For this review, take the finished solid that the model builds, in its own axes (mm). Face numbers are marked on the shaded views. A direction names the side the tool comes from. Round coordinates to 2 decimals unless told otherwise and drop trailing zeros. Write each loop counter-clockwise with the first axis right and the second up, starting at its lowest first coordinate (ties: lowest second). Pieces come first, ordered by that corner, then holes. Notation, with made-up numbers: (14.25, -18) -> (23.25, -18) arc R6 cw to (23.25, -7) -> close; hole circle Ø2 at (-24, -4). An arc over 180 degrees is marked (long way). Answer in a Markdown table with one row per item.
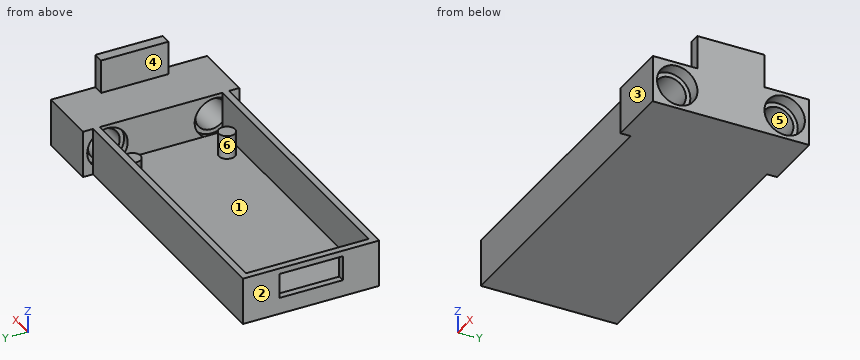
from build123d import *

# Parameters (mm, degrees)
SKETCH1_W              = 39
SKETCH1_H              = 20.2
BOSS_EXTRUDE1_DEPTH    = 7
SKETCH2_W              = 38
SKETCH2_H              = 18.2
CUT_EXTRUDE1_DEPTH     = 6
SKETCH3_R              = 1.2
SPUNT_DEPTH            = 3.5
SKETCH5_W              = 3.7
SKETCH5_H              = 9.4
USBC_DEPTH             = 22
ROZSIRENI_DRZAKU_DEPTH = 3
SKETCH7_W              = 7
SKETCH7_H              = 23.2
DRZAK_DEPTH            = 9
SKETCH8_R              = 2.35
ZAKLADNI_DIRA_DEPTH    = 9
SKETCH9_R              = 3
CUT_EXTRUDE4_DEPTH     = 2
SKETCH11_R             = 3
CUT_EXTRUDE5_DEPTH     = 1
SKETCH10_W             = 1.6
SKETCH10_H             = 10
PODSTAVA_DEPTH         = 5


with BuildPart() as part:
    # Sketch1 → Boss-Extrude1 (new body)
    with BuildSketch(Plane.XY):
        Rectangle(SKETCH1_W, SKETCH1_H)
    extrude(amount=BOSS_EXTRUDE1_DEPTH)

    # Sketch2 → Cut-Extrude1 (cut)
    with BuildSketch(Plane.XY.offset(7)):
        with Locations((0.5, 0)):
            Rectangle(SKETCH2_W, SKETCH2_H)
    extrude(amount=-CUT_EXTRUDE1_DEPTH, mode=Mode.SUBTRACT)

    # Sketch3 → spunt (add)
    with BuildSketch(Plane.XY.offset(1)):
        with Locations((17.3, -7)):
            Circle(SKETCH3_R)
        with Locations((17.3, 7)):
            Circle(SKETCH3_R)
    extrude(amount=SPUNT_DEPTH)

    # Sketch5 → usbc (cut)
    with BuildSketch(Plane(origin=(-18.5, 0, 0), x_dir=(0, 0, -1), z_dir=(1, 0, 0))):
        with Locations((-4.3, 0)):
            Rectangle(SKETCH5_W, SKETCH5_H)
    extrude(amount=-USBC_DEPTH, mode=Mode.SUBTRACT)

    # Sketch6 → rozsireni drzaku (add)
    with BuildSketch(Plane(origin=(19.5, 0, 0), x_dir=(0, 0, -1), z_dir=(1, 0, 0))):
        Polygon((-7, -10.1), (0, -10.1), (0, 10.1), (-7, 10.1), (-7, 9.1), (-1, 9.1), (-1, -9.1), (-7, -9.1), align=None)
    extrude(amount=ROZSIRENI_DRZAKU_DEPTH)

    # Sketch7 → drzak (add)
    with BuildSketch(Plane(origin=(22.5, 0, 0), x_dir=(0, 0, -1), z_dir=(1, 0, 0))):
        with Locations((-3.5, 0)):
            Rectangle(SKETCH7_W, SKETCH7_H)
    extrude(amount=DRZAK_DEPTH)

    # Sketch8 → zakladni dira (cut)
    with BuildSketch(Plane(origin=(31.5, 0, 0), x_dir=(0, 0, -1), z_dir=(1, 0, 0))):
        with Locations((-3.5, 7.97)):
            Circle(SKETCH8_R)
        with Locations((-3.5, -7.97)):
            Circle(SKETCH8_R)
    extrude(amount=-ZAKLADNI_DIRA_DEPTH, mode=Mode.SUBTRACT)

    # Sketch9 → Cut-Extrude4 (cut)
    with BuildSketch(Plane(origin=(31.5, 0, 0), x_dir=(0, 0, -1), z_dir=(1, 0, 0))):
        with Locations((-3.5, 7.97)):
            Circle(SKETCH9_R)
        with Locations((-3.5, -7.97)):
            Circle(SKETCH9_R)
    extrude(amount=-CUT_EXTRUDE4_DEPTH, mode=Mode.SUBTRACT)

    # Sketch11 → Cut-Extrude5 (cut)
    with BuildSketch(Plane.ZY.offset(-22.5)):
        with Locations((3.5, -7.97)):
            Circle(SKETCH11_R)
        with Locations((3.5, 7.97)):
            Circle(SKETCH11_R)
    extrude(amount=-CUT_EXTRUDE5_DEPTH, mode=Mode.SUBTRACT)

    # Sketch10 → podstava (add)
    with BuildSketch(Plane.XY.offset(7)):
        with Locations((30.7, 0)):
            Rectangle(SKETCH10_W, SKETCH10_H)
    extrude(amount=PODSTAVA_DEPTH)


solid = part.part
1) For the marked faces 4, 5 and 6, list the 3-axis set-ups (+Z, -Z, +X, -X, +Y, -Y) from which the entire face can be reached by the end or side of a thin tool; tool diameter is ignored.
Solved:
| item | result |
|---|---|
| face 4 | +Z, -X, +Y, -Y |
| face 5 | +X |
| face 6 | +Z |
2) Consider section B-B on x = 17.3. State the section outline as (y, z) points, then the cut area to 3 significant figures.
Solved:
| item | result |
|---|---|
| outline | (-10.1, 0) -> (10.1, 0) -> (10.1, 7) -> (9.1, 7) -> (9.1, 1) -> (8.2, 1) -> (8.2, 4.5) -> (5.8, 4.5) -> (5.8, 1) -> (-5.8, 1) -> (-5.8, 4.5) -> (-8.2, 4.5) -> (-8.2, 1) -> (-9.1, 1) -> (-9.1, 7) -> (-10.1, 7) -> close |
| area | 49.0 mm² |
3) For line 1 (Y direction, x = 26.2, z = 3.5); line 2 (X direction, y = 4.25, z = 1.25); line 3 (Z direction, x = 22.8, y = -7.97), list the stretches that pass through material, from the lowest coordinate up. Write a range as [from, to].
Solved:
| item | result |
|---|---|
| line 1 | [-11.6, -10.32], [-5.62, 5.62], [10.32, 11.6] |
| line 2 | [-19.5, -18.5], [22.5, 31.5] |
| line 3 | [0, 0.5], [6.5, 7] |
4) Consider section C-C on z = 3.5. State how many separate pieces and enclosed holes the cut face has, then the cut area to 3 significant figures.
Solved:
| item | result |
|---|---|
| separate pieces | 7 |
| enclosed holes | 0 |
| area | 218 mm² |
5) Mouldability with a two-part tool opening along X and no side actions: class the marked faces 1, 2 and 3 as pulls with the +X half, pulls with the -X half, needs draft (parallel to the pull), parting line crosses it, or undercut.
Solved:
| item | result |
|---|---|
| face 1 | undercut |
| face 2 | pulls with the -X half |
| face 3 | needs draft |
6) Consider section D-D on y = 7. State the section outline as (x, z) points, then the cut area to 3 significant figures.
Solved:
| item | result |
|---|---|
| outline | (-19.5, 0) -> (31.5, 0) -> (31.5, 0.66) -> (29.5, 0.66) -> (29.5, 1.36) -> (23.5, 1.36) -> (23.5, 0.66) -> (22.5, 0.66) -> (22.5, 1) -> (18.5, 1) -> (18.5, 4.5) -> (16.1, 4.5) -> (16.1, 1) -> (-18.5, 1) -> (-18.5, 7) -> (-19.5, 7) -> close; (22.5, 6.34) -> (23.5, 6.34) -> (23.5, 5.64) -> (29.5, 5.64) -> (29.5, 6.34) -> (31.5, 6.34) -> (31.5, 7) -> (22.5, 7) -> close |
| area | 76.7 mm² |
7) Consider section A-A on y = -0.75. State the section outline as (x, z) points.
Solved:
| item | result |
|---|---|
| outline | (-19.5, 0) -> (31.5, 0) -> (31.5, 12) -> (29.9, 12) -> (29.9, 7) -> (22.5, 7) -> (22.5, 1) -> (-18.5, 1) -> (-18.5, 2.45) -> (-19.5, 2.45) -> close; (-19.5, 6.15) -> (-18.5, 6.15) -> (-18.5, 7) -> (-19.5, 7) -> close |
8) Clearance check with flat-ended pins moving along their axes: pin 1 Ø5 at (x, y) = (-7.5, 6.5) entering from +Z; pin 2 Ø1.2 at (x, y) = (17, 7.5) entering from +Z; pin 3 Ø3 at (x, z) = (3, 5) entering from -Y. State where each tip first meets the part, or that it passes through.
Solved:
| item | result |
|---|---|
| pin 1 | z = 1 |
| pin 2 | z = 4.5 |
| pin 3 | y = -10.1 |
